The figure shows three views and two pictorial views of one solid part (mm, origin at its lowest corner). Answer the questions. Round coordinates to 2 decimals unless told otherwise and drop trailing zeros. Write each loop counter-clockwise with the first axis right and the second up, starting at its lowest first coordinate (ties: lowest second). Pieces come first, ordered by that corner, then holes. Notation, with made-up numbers: (-27, -33) -> (-5, -33) arc R17 cw to (-5, -1) -> close; hole circle Ø4 at (-15, 60). An arc over 180 degrees is marked (long way). One line per item, written item: value.
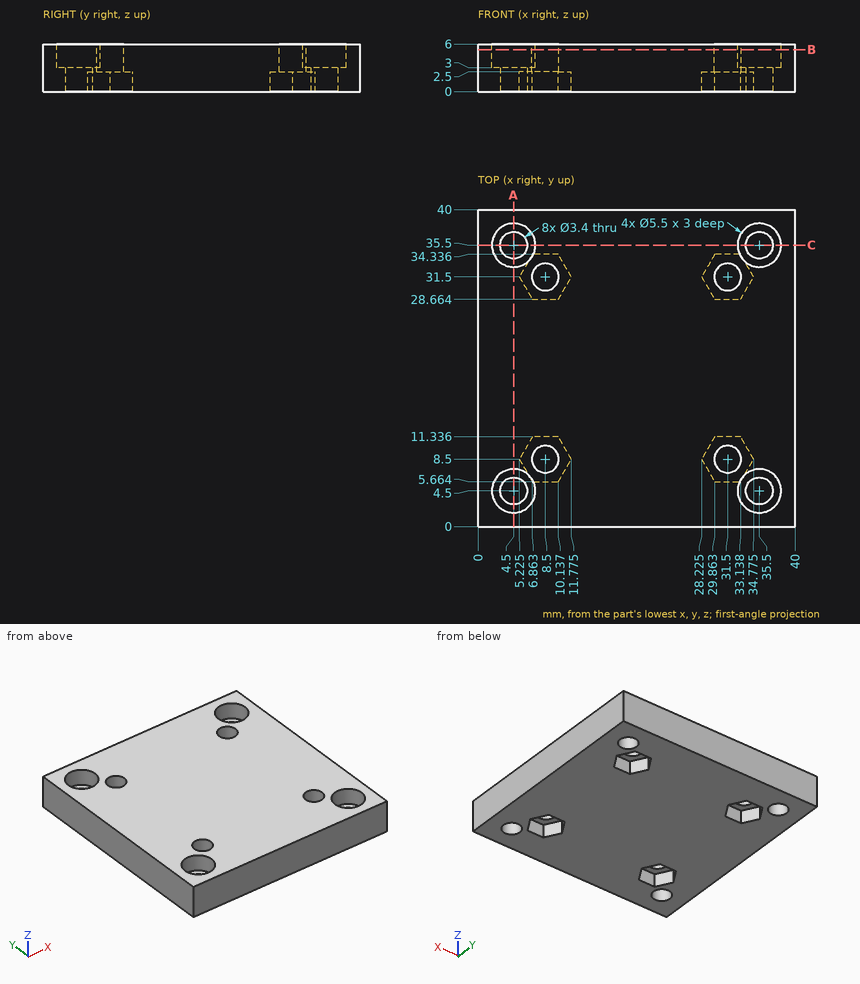
(1) Flat-ended cylindrical pins translate along their axes: pin 1 Ø3 at (x, y) = (35, 5.5) entering from +Z; pin 2 Ø1 at (x, y) = (10, 9) entering from -Z. Find the tip coordinate at first contact, or state that the pin passes through.
Reported:
pin 1: stops at z = 3
pin 2: stops at z = 2.5
(2) Find section B-B on z = 5.3. Give the number of separate pieces and of enclosed holes in the cut face, plus the area to 3 significant figures.
Reported:
separate pieces: 1
enclosed holes: 8
area: 1,470 mm2
(3) Find section A-A on x = 4.5. Give the vertices of the cut face in (y, z).
Reported:
outline: (0, 0) -> (2.8, 0) -> (2.8, 3) -> (1.75, 3) -> (1.75, 6) -> (0, 6) -> close; (6.2, 0) -> (33.8, 0) -> (33.8, 3) -> (32.75, 3) -> (32.75, 6) -> (7.25, 6) -> (7.25, 3) -> (6.2, 3) -> close; (37.2, 0) -> (40, 0) -> (40, 6) -> (38.25, 6) -> (38.25, 3) -> (37.2, 3) -> close
(4) Consider probe 1 along Y at (x, z) = (35.5, 2); probe 2 along Y at (x, z) = (33, 2.2); probe 3 along X at (y, z) = (31.5, 4.8). Determine where each line is inside the solid, lowest interval first.
Reported:
probe 1: y = 0 to 2.8, 6.2 to 33.8, 37.2 to 40
probe 2: y = 0 to 5.66, 11.34 to 28.66, 34.34 to 40
probe 3: x = 0 to 6.8, 10.2 to 29.8, 33.2 to 40
